For this review, use the dimensioned drawing (mm, ordinates from the lowest corner) and the shaded views. A direction names the side the tool comes from. Coordinates: 2 decimals unless noted, no trailing zeros. Loops run counter-clockwise (first coordinate to the right, second up) from the corner with the lowest first, then second, coordinate; pieces in that order, holes last. Notation, with made-up numbers: (85.25, -14.75) - (141.25, -14.75) arc R25 cw to (141.25, -1.75) - close; hole circle Ø11 at (-25.75, 82.25). An arc over 180 degrees is marked (long way). Answer in a Markdown table with one row per item. Add a question column.
(1) We need section D-D, the plane y = 24. Write out the cut boundary in (x, z) (1 decimal), plus the area to 3 significant figures.
(2) Clearance check with flat-ended pins moving along their axes: pin 1 (0.9 mm diameter, centred on y = 2, z = 1.5, fed in from -X); pin 2 (1.6 mm diameter, centred on x = 4.04, y = 23.53, fed in from +Z); pin 3 (0.9 mm diameter, centred on x = 7, z = 2, fed in from -Y). State where each tip first meets the part, or that it passes through.
(3) We need section A-A, the plane y = 4.5. Write out the cut boundary in (x, z).
(4) We need section C-C, the plane x = 9.5. Write out the cut boundary in (y, z).
(5) The part is to be moulded in two halves that separate along X. For the marked faces 1, 2, 3 and 4, say which applies: released by +X, released by -X, zero draft, split by the parting line, or undercut.
(6) For the marked faces 5 and 6, list the 3-axis set-ups (+Z, -Z, +X, -X, +Y, -Y) from which the entire face can be reached by the end or side of a thin tool; tool diameter is ignored.
(7) To check wall thickness, follow L1, parallel to Y at x = 10.5, z = 2.5; L2, parallel to X at y = 4.5, z = 2; L3, parallel to Y at x = 4, z = 1.9. State the ranges of each line that lie inside material, in increasing order. Write a range as [from, to].
(8) We need section B-B, the plane z = 1.1. Write out the cut boundary in (x, y).
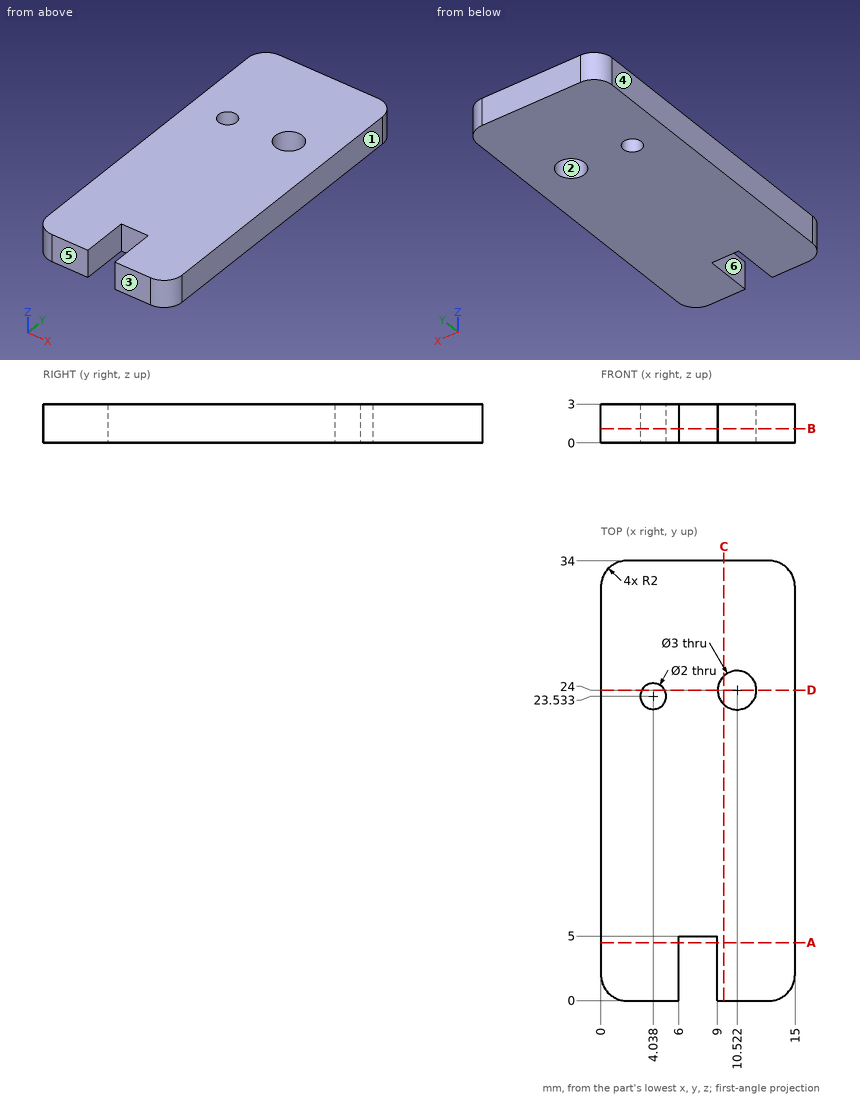
Responses:
| question | item | result |
|---|---|---|
| 1 | outline | (0, 0) - (3.2, 0) - (3.2, 3) - (0, 3) - close; (4.9, 0) - (9, 0) - (9, 3) - (4.9, 3) - close; (12, 0) - (15, 0) - (15, 3) - (12, 3) - close |
| 1 | area | 30.7 mm2 |
| 2 | pin 1 | stops at x = 0 |
| 2 | pin 2 | passes through |
| 2 | pin 3 | stops at y = 5 |
| 3 | outline | (0, 0) - (6, 0) - (6, 3) - (0, 3) - close; (9, 0) - (15, 0) - (15, 3) - (9, 3) - close |
| 4 | outline | (0, 0) - (22.9, 0) - (22.9, 3) - (0, 3) - close; (25.1, 0) - (34, 0) - (34, 3) - (25.1, 3) - close |
| 5 | face 1 | released by +X |
| 5 | face 2 | undercut |
| 5 | face 3 | zero draft |
| 5 | face 4 | released by -X |
| 6 | face 5 | +Z, -Z, +X, -X, -Y |
| 6 | face 6 | +Z, -Z, -Y |
| 7 | L1 | y = [0, 22.5], [25.5, 34] |
| 7 | L2 | x = [0, 6], [9, 15] |
| 7 | L3 | y = [0, 22.53], [24.53, 34] |
| 8 | outline | (0, 2) arc R2 ccw to (2, 0) - (6, 0) - (6, 5) - (9, 5) - (9, 0) - (13, 0) arc R2 ccw to (15, 2) - (15, 32) arc R2 ccw to (13, 34) - (2, 34) arc R2 ccw to (0, 32) - close; hole circle Ø2 at (4.04, 23.53); hole circle Ø3 at (10.52, 24) |
